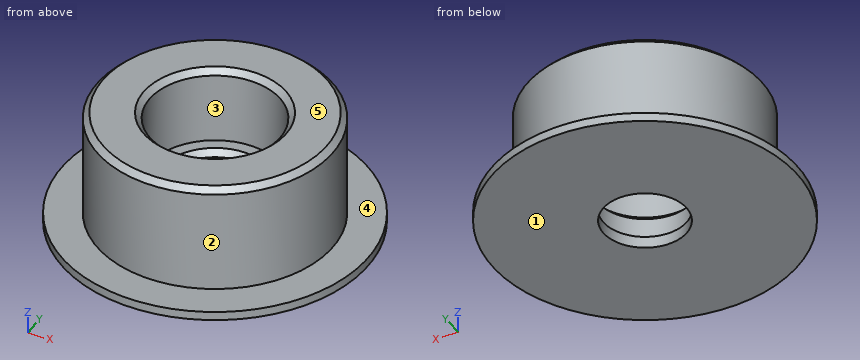
from build123d import *

# Parameters (mm, degrees)
F0_R     = 8.1
F0_R_2   = 7.1
F1_DEPTH = 2
F0_R_3   = 11.1
F2_DEPTH = 7
F0_R_4   = 20
F3_DEPTH = 20
F0_R_5   = 26
F4_DEPTH = 1.5
F5_SIZE  = 1


with BuildPart() as f1:
    # F0 (on Top) → F1 (new body)
    with BuildSketch(Plane.XY):
        Circle(F0_R)
        Circle(F0_R_2, mode=Mode.SUBTRACT)
    extrude(amount=F1_DEPTH)

    # F0 (on Top) → F2 (join)
    with BuildSketch(Plane.XY):
        Circle(F0_R_3)
        Circle(F0_R, mode=Mode.SUBTRACT)
    extrude(amount=F2_DEPTH)

    # F0 (on Top) → F3 (join)
    with BuildSketch(Plane.XY):
        Circle(F0_R_4)
        Circle(F0_R_3, mode=Mode.SUBTRACT)
    extrude(amount=F3_DEPTH)

    # F0 (on Top) → F4 (join)
    with BuildSketch(Plane.XY):
        Circle(F0_R_5)
        Circle(F0_R_4, mode=Mode.SUBTRACT)
    extrude(amount=F4_DEPTH)

    # F5
    f5_edges = [f1.edges().sort_by_distance(p)[0] for p in [
        (-20, 0, 20),
        (-11.1, 0, 20),
        (-8.1, 0, 7),
    ]]
    chamfer(f5_edges, length=F5_SIZE)


solid = f1.part
Part model, mm, in its own coordinate system. Face numbers are marked on the shaded views. A direction names the side the tool comes from. Give positions to 0.01 mm unless a question says otherwise; leave off trailing zeros. Loops run counter-clockwise (first coordinate to the right, second up) from the corner with the lowest first, then second, coordinate; pieces in that order, holes last.
(1) Drill centre lines: line 1 along Y through (x, z) = (0, 4.15); line 2 along Y through (x, z) = (0, 15); line 3 along Z through (x, y) = (-1, -23.5). Where is each one in solid material? Low to high.
Return value:
line 1: y = -20 to -8.1, 8.1 to 20
line 2: y = -20 to -11.1, 11.1 to 20
line 3: z = 0 to 1.5
(2) Band-saw the part on D-D (y = 21.5). Write the cut outline in (x, z).
Return value:
outline: (-14.62, 0) - (14.62, 0) - (14.62, 1.5) - (-14.62, 1.5) - close
(3) 3-axis set-ups, long thin cutter, end or side, ignore diameter. For the marked faces 4 and 5: which of +Z, -Z, +X, -X, +Y, -Y reach the whole face in a straight line?
Return value:
face 4: +Z
face 5: +Z, +X, -X, +Y, -Y
(4) Pull direction X, two halves, no side cores. Call the marked faces 1, 2 and 3: pulls with the +X half, pulls with the -X half, needs draft (parallel to the pull), parting line crosses it, or undercut.
Return value:
face 1: needs draft
face 2: parting line crosses it
face 3: undercut
(5) Band-saw the part on C-C (z = 13.75). Write the cut outline in (x, y).
Return value:
outline: circle Ø40 at (0, 0); hole circle Ø22.2 at (0, 0)
(6) Pin check, flat tips, straight feed: pin 1 (13.5 mm diameter, centred on x = 0, y = 0, fed in from -Z); pin 2 (22.5 mm diameter, centred on x = 0, y = 0, fed in from -Z); pin 3 (12 mm diameter, centred on x = -2, z = 12, fed in from +Y); pin 4 (8 mm diameter, centred on y = -5, z = 13, fed in from +X) (3 decimals). Stop position of each tip, or through.
Return value:
pin 1: passes through
pin 2: stops at z = 0
pin 3: stops at y = 20
pin 4: stops at x = 19.975
(7) Band-saw the part on A-A (y = 0). Write the cut outline in (x, z).
Return value:
outline: (-26, 0) - (-7.1, 0) - (-7.1, 2) - (-8.1, 2) - (-8.1, 6) - (-9.1, 7) - (-11.1, 7) - (-11.1, 19) - (-12.1, 20) - (-19, 20) - (-20, 19) - (-20, 1.5) - (-26, 1.5) - close; (7.1, 0) - (26, 0) - (26, 1.5) - (20, 1.5) - (20, 19) - (19, 20) - (12.1, 20) - (11.1, 19) - (11.1, 7) - (9.1, 7) - (8.1, 6) - (8.1, 2) - (7.1, 2) - close
